Geometry: final body of the model. Coordinates: model frame, mm. Coordinates: 2 decimals unless noted, no trailing zeros. Write each loop counter-clockwise with the first axis right and the second up, starting at its lowest first coordinate (ties: lowest second). Pieces come first, ordered by that corner, then holes. Notation, with made-up numbers: (29, -2.75) - (43, -2.75) arc R19 ccw to (43, 29.25) - close; hole circle Ø2 at (-37, -7). An arc over 180 degrees is marked (long way). Answer as a JSON object with one key per item and string values. Group by question number.
Item 1: First-contact query: pin 1 Ø4 at (x, y) = (86, -238) entering from +Z; pin 2 Ø2.5 at (y, z) = (295, 4) entering from -X; pin 3 Ø4 at (y, z) = (-22.5, 2.5) entering from -X; pin 4 Ø3 at (x, z) = (-243, 8) entering from -Y. Flat tips, straight axial feed; report the tip coordinate or a pass-through.
Item 2: Line query: line 1 along X through (y, z) = (-238, 8); line 2 along Y through (x, z) = (-86, 5); line 3 along Y through (x, z) = (-74, 6.75). Output: solid intervals per line, ascending. Write a range as from..to.
Item 3: Section C-C on y = 9. Return loops of the section in (x, z), and give its area (3 significant figures).
Item 4: Section B-B on x = 158. Return loops of the section in (y, z), and give its area (3 significant figures).
Item 5: Section A-A on z = 5. Return loops of the section in (x, y), and give its area (3 significant figures).
```python
from build123d import *

# Parameters (mm, degrees)
SKETCH1_W           = 400
SKETCH1_H           = 500
BOSS_EXTRUDE1_DEPTH = 10
SKETCH2_R           = 2.5
CUT_EXTRUDE1_DEPTH  = 321.312347561
SKETCH3_W           = 10
SKETCH3_H           = 10
BOSS_EXTRUDE2_DEPTH = 50
SKETCH4_W           = 10
SKETCH4_H           = 10
BOSS_EXTRUDE3_DEPTH = 400
SKETCH5_R           = 2.5
CUT_EXTRUDE2_DEPTH  = 10


with BuildPart() as part:
    # Sketch1 → Boss-Extrude1 (new body)
    with BuildSketch(Plane.XY):
        Rectangle(SKETCH1_W, SKETCH1_H)
    extrude(amount=BOSS_EXTRUDE1_DEPTH)

    # Sketch2 → Cut-Extrude1 (cut, through all)
    with BuildSketch(Plane.XY.offset(10)):
        with Locations((-86, -238)):
            Circle(SKETCH2_R)
        with Locations((-60, -225)):
            Circle(SKETCH2_R)
        with Locations((-34, -238)):
            Circle(SKETCH2_R)
        with Locations((34, -238)):
            Circle(SKETCH2_R)
        with Locations((60, -225)):
            Circle(SKETCH2_R)
        with Locations((86, -238)):
            Circle(SKETCH2_R)
    extrude(amount=-CUT_EXTRUDE1_DEPTH, mode=Mode.SUBTRACT)

    # Sketch3 → Boss-Extrude2 (add)
    with BuildSketch(Plane(origin=(0, 250, 0), x_dir=(1, 0, 0), z_dir=(0, 1, 0))):
        with Locations((0, -5)):
            Rectangle(SKETCH3_W, SKETCH3_H)
    extrude(amount=BOSS_EXTRUDE2_DEPTH)

    # Sketch4 → Boss-Extrude3 (add)
    with BuildSketch(Plane.ZY.offset(5)):
        with Locations((5, 295)):
            Rectangle(SKETCH4_W, SKETCH4_H)
    extrude(amount=BOSS_EXTRUDE3_DEPTH)

    # Sketch5 → Cut-Extrude2 (cut)
    with BuildSketch(Plane.ZY.offset(405)):
        with Locations(Location((5, 295, 0), (0, 0, 270))):
            Circle(SKETCH5_R)
    extrude(amount=-CUT_EXTRUDE2_DEPTH, mode=Mode.SUBTRACT)


solid = part.part
```
Checks:
{
 "1": {"pin 1": "through", "pin 2": "x = -395", "pin 3": "x = -200", "pin 4": "y = 290"},
 "2": {"line 1": "-200..-88.5, -83.5..-36.5, -31.5..31.5, 36.5..83.5, 88.5..200", "line 2": "-250..-240.5, -235.5..250, 290..300", "line 3": "-250..250, 290..300"},
 "3": {"outline": "(-200, 0) - (200, 0) - (200, 10) - (-200, 10) - close", "area": "4,000 mm^2"},
 "4": {"outline": "(-250, 0) - (250, 0) - (250, 10) - (-250, 10) - close", "area": "5,000 mm^2"},
 "5": {"outline": "(-405, 290) - (-5, 290) - (-5, 250) - (-200, 250) - (-200, -250) - (200, -250) - (200, 250) - (5, 250) - (5, 300) - (-405, 300) - (-405, 297.5) - (-395, 297.5) - (-395, 292.5) - (-405, 292.5) - close; hole circle Ø5 at (-86, -238); hole circle Ø5 at (-60, -225); hole circle Ø5 at (-34, -238); hole circle Ø5 at (34, -238); hole circle Ø5 at (60, -225); hole circle Ø5 at (86, -238)", "area": "204,000 mm^2"}
}
